Could you check a few things on this model? Use its own coordinates, in mm. Face numbers are marked on the shaded views. A direction names the side the tool comes from. Give positions to 0.01 mm unless a question says otherwise; leave off trailing zeros. Loops run counter-clockwise (first coordinate to the right, second up) from the corner with the lowest first, then second, coordinate; pieces in that order, holes last. Notation, with made-up numbers: (-38, 41.25) -> (2, 41.25) arc R29 ccw to (2, 66.25) -> close; hole circle Ø6 at (56, 76). An arc over 180 degrees is marked (long way). Write item = value, one per line. Start each with the question number.
1) I want a section at B-B (z = 0). List the corners of the cut face in (x, y) for me.
2) I want a section at A-A (y = 17.25). List the corners of the cut face in (x, z) for me, and give its area (3 significant figures).
3) I want a section at C-C (y = 13). List the corners of the cut face in (x, z) for me, and give its area (3 significant figures).
4) I'm going to push flat-ended pins straight in: pin 1 Ø1 at (y, z) = (4, -1.5) entering from -X; pin 2 Ø3 at (y, z) = (12, -1.5) entering from +X; pin 3 Ø1 at (x, y) = (1, 15.5) entering from -Z. Where does each tip first touch, or does it pass through?
5) I need wall thicknesses on probe 1 along Z at (x, y) = (-1.5, 5.5); probe 2 along X at (y, z) = (16, -1.25); probe 3 along Y at (x, z) = (-0.25, -1). Which ranges of each line are inside material? Lowest first, please. Write a range as from..to.
6) I want a section at D-D (x = -3). List the corners of the cut face in (y, z) for me.
7) On a 3-axis mill with a long thin cutter (end or side, diameter ignored), from which of +Z, -Z, +X, -X, +Y, -Y can I reach the whole of each face in a straight line? I mean the marked faces 1, 2 and 3. Say none if no direction works.
8) If we mould it in two halves opening along Z, with no side actions, what happens to the marked faces 4, 5 and 6? For each: +Z half, -Z half, draft (parallel to the pull), parting line (faces both ways), or undercut.
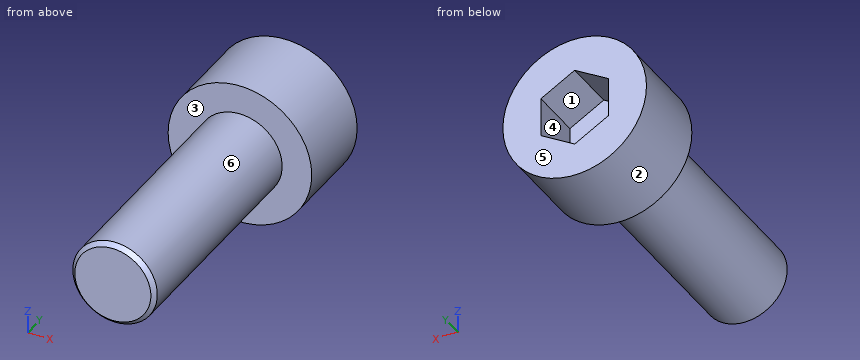
Autodesk Inventor part; units mm, degrees
ref_plane "YZ Plane" through (0, 0, 0) normal (1, 0, 0) x (0, 1, 0)
ref_plane "XZ Plane" through (0, 0, 0) normal (0, 1, 0) x (-1, 0, 0)
ref_plane "XY Plane" through (0, 0, 0) normal (0, 0, 1) x (1, 0, 0)
sketch "Sketch1" plane through (0, 0, 0) normal (0, 1, 0) x (-1, 0, 0)
  circle A0 centre (0, 0) radius 2.5
  dimension "d0" = 5
extrude "Extrusion1" add sketch "Sketch1" along normal blind 14
sketch "Sketch2" plane through (0, 14, 0) normal (0, 1, 0) x (1, 0, 0)
  circle A0 centre (0, 0) radius 2.5
  circle A1 centre (0, 0) radius 4.25
  dimension "d3" = 8.5
extrude "Extrusion2" add sketch "Sketch2" along normal blind 5 contours A0 | A1
sketch "Sketch3" plane through (0, 19, 0) normal (0, 1, 0) x (1, 0, 0)
  circle A0 centre (0, 0) radius 4.25
  line L0 (0, 2.3094) -> (2, 1.1547)
  line L1 (2, 1.1547) -> (2, -1.1547)
  line L2 (2, -1.1547) -> (0, -2.3094)
  line L3 (0, -2.3094) -> (-2, -1.1547)
  line L4 (-2, -1.1547) -> (-2, 1.1547)
  line L5 (-2, 1.1547) -> (0, 2.3094)
  dimension "d6" = 2
extrude "Extrusion3" cut sketch "Sketch3" against normal blind 3.2 contours L0 L1 L2 L3 L4 L5
thread "Thread1"
chamfer "Chamfer1" distance 0.25 angle 45 1 edges at (2.5, 0, 0)
properties part number "M5x14SHCS" material "Stainless Steel"
Answer list:
q1.outline = (-4.25, 14) -> (-2.5, 14) -> (-2.5, 0.25) -> (-2.25, 0) -> (2.25, 0) -> (2.5, 0.25) -> (2.5, 14) -> (4.25, 14) -> (4.25, 19) -> (2, 19) -> (2, 15.8) -> (-2, 15.8) -> (-2, 19) -> (-4.25, 19) -> close
q2.outline = circle Ø8.5 at (0, 0); hole (-2, -1.15) -> (0, -2.31) -> (2, -1.15) -> (2, 1.15) -> (0, 2.31) -> (-2, 1.15) -> close
q2.area = 42.9 mm^2
q3.outline = circle Ø5 at (0, 0)
q3.area = 19.6 mm^2
q4.pin_1 = -2.29
q4.pin_2 = 2.5
q4.pin_3 = -4.22
q5.probe_1 = -2..2
q5.probe_2 = -4.06..-1.83, 1.83..4.06
q5.probe_3 = 0..15.8
q6.outline = (14, -3.01) -> (19, -3.01) -> (19, 3.01) -> (14, 3.01) -> close
q7.face_1 = +Y
q7.face_2 = +Y, -Y
q7.face_3 = -Y
q8.face_4 = undercut
q8.face_5 = draft
q8.face_6 = parting line
